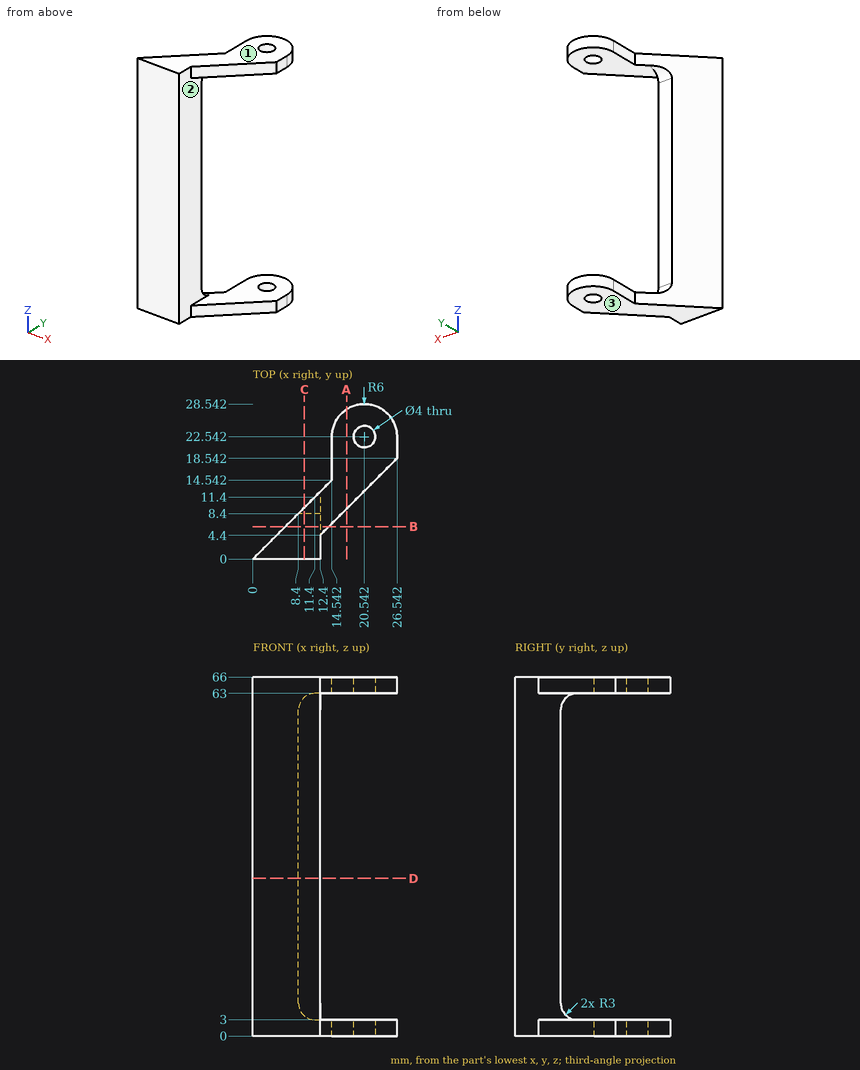
Input: dimensioned drawing with shaded views. Units: mm. Origin: part minimum x, y, z. Give positions to 0.01 mm unless a question says otherwise; leave off trailing zeros. Order: outer loops, then holes, each group sorted by start corner. A loop starts at its lowest first (then second) coordinate and runs counter-clockwise, first axis right, second up.
(1) Section query C-C (x = 9.5). Return the cut outline in (y, z), plus the area to 3 significant figures.
(2) Contact query for flat-ended pins moving along their axis: P1, Ø12, axis at x = 20.5, y = 12, coming from the +Z side; P2, Ø4.5, axis at x = 9.5, z = 20.5, coming from the +Y side; P3, Ø1, axis at y = 3.5, z = 33, coming from the -X side; P4, Ø12.5, axis at y = 4, z = 32, coming from the +X side. Output: stop coordinate, or through.
(3) Pull-direction query (Z, two-part tool) for the marked faces 1, 2 and 3; classes: +Z half, -Z half, draft (parallel to the pull), parting line (faces both ways), or undercut.
(4) Section query B-B (y = 6). Return the cut outline in (x, z), plus the area to 3 significant figures.
(5) Material intervals for line 1 along Z through (x, y) = (24.75, 24); line 2 along X through (y, z) = (3, 5); line 3 along Y through (x, z) = (11, 6), sorted ascending.
(6) Section query A-A (x = 17.25). Return the cut outline in (y, z), plus the area to 3 significant figures.
(7) Section query D-D (z = 29). Return the cut outline in (x, y).
Outcome:
1. outline: (0, 0) - (9.5, 0) - (9.5, 3.68) arc R3 cw to (8.4, 6) - (8.4, 60) arc R3 cw to (9.5, 62.32) - (9.5, 66) - (0, 66) - close
1. area: 564 mm2
2. P1: stops at z = 66
2. P2: stops at y = 8.4
2. P3: stops at x = 3
2. P4: stops at x = 12.4
3. face 1: +Z half
3. face 2: undercut
3. face 3: -Z half
4. outline: (6, 0) - (14, 0) - (14, 3) - (12.4, 3) - (12.4, 63) - (14, 63) - (14, 66) - (6, 66) - close
4. area: 432 mm2
5. line 1: z = 0 to 3, 63 to 66
5. line 2: x = 3 to 12.4
5. line 3: y = 0 to 8.4
6. outline: (9.25, 0) - (27.56, 0) - (27.56, 3) - (9.25, 3) - close; (9.25, 63) - (27.56, 63) - (27.56, 66) - (9.25, 66) - close
6. area: 110 mm2
7. outline: (0, 0) - (12.4, 0) - (12.4, 8.4) - (8.4, 8.4) - close
